Can you work these out from the model? Positions are in its coordinate system, mm. Give positions to 0.01 mm unless a question says otherwise; leave off trailing zeros. Write each loop counter-clockwise with the first axis right and the second up, starting at its lowest first coordinate (ties: lowest second). Pieces come first, ordered by that corner, then holes. Notation, with made-up numbers: (50.5, 19) -> (107.5, 19) arc R31 ccw to (107.5, 49) -> close; hole circle Ø2 at (48.5, 44.5). An arc over 180 degrees is marked (long way). One line per item, written item: value.
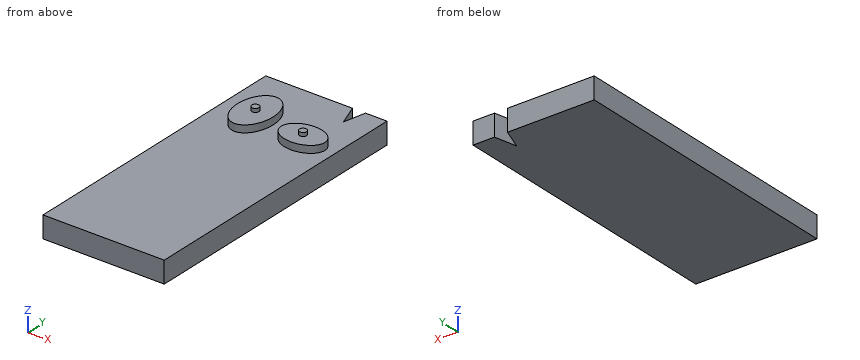
from build123d import *

# Parameters (mm, degrees)
F1_DEPTH = 3
F0_R     = 0.5
F2_DEPTH = 4
F3_DEPTH = 4.5


with BuildPart() as f1:
    # F0 (on Top) → F1 (new body)
    with BuildSketch(Plane.XY):
        Polygon((-42.22717, 54.8594), (-54.246616, 54.8594), (-54.246616, 14.957247), (-37.451323, 14.957247), (-37.451323, 54.8594), (-40.430126, 54.8594), (-41.114714, 51.767185), align=None)
        with BuildLine():
            add(Edge.make_bspline(
                [(-49.261443, 42.794443), (-44.9895, 42.794443), (-47.125472, 48.428944), (-49.261443, 54.063445), (-51.397415, 48.428944), (-53.533386, 42.794443), (-49.261443, 42.794443)],
                knots=[0, 0, 0, 2.094395, 2.094395, 4.18879, 4.18879, 6.283185, 6.283185, 6.283185], degree=2, weights=[1, 0.5, 1, 0.5, 1, 0.5, 1]))
        make_face(mode=Mode.SUBTRACT)
        with BuildLine():
            add(Edge.make_bspline(
                [(-38.755624, 45.423176), (-38.755624, 49.162015), (-43.297707, 47.292595), (-47.83979, 45.423176), (-43.297707, 43.553757), (-38.755624, 41.684338), (-38.755624, 45.423176)],
                knots=[0, 0, 0, 2.094395, 2.094395, 4.18879, 4.18879, 6.283185, 6.283185, 6.283185], degree=2, weights=[1, 0.5, 1, 0.5, 1, 0.5, 1]))
        make_face(mode=Mode.SUBTRACT)
    extrude(amount=F1_DEPTH)

    # F0 (on Top) → F2 (join)
    with BuildSketch(Plane.XY):
        with BuildLine():
            add(Edge.make_bspline(
                [(-49.261443, 42.794443), (-44.9895, 42.794443), (-47.125472, 48.428944), (-49.261443, 54.063445), (-51.397415, 48.428944), (-53.533386, 42.794443), (-49.261443, 42.794443)],
                knots=[0, 0, 0, 2.094395, 2.094395, 4.18879, 4.18879, 6.283185, 6.283185, 6.283185], degree=2, weights=[1, 0.5, 1, 0.5, 1, 0.5, 1]))
        make_face()
        with Locations((-49.261443, 46.550777)):
            Circle(F0_R, mode=Mode.SUBTRACT)
        with BuildLine():
            add(Edge.make_bspline(
                [(-38.755624, 45.423176), (-38.755624, 49.162015), (-43.297707, 47.292595), (-47.83979, 45.423176), (-43.297707, 43.553757), (-38.755624, 41.684338), (-38.755624, 45.423176)],
                knots=[0, 0, 0, 2.094395, 2.094395, 4.18879, 4.18879, 6.283185, 6.283185, 6.283185], degree=2, weights=[1, 0.5, 1, 0.5, 1, 0.5, 1]))
        make_face()
        with Locations((-41.783679, 45.423176)):
            Circle(F0_R, mode=Mode.SUBTRACT)
    extrude(amount=F2_DEPTH)

    # F0 (on Top) → F3 (join)
    with BuildSketch(Plane.XY):
        with Locations((-49.261443, 46.550777)):
            Circle(F0_R)
        with Locations((-41.783679, 45.423176)):
            Circle(F0_R)
    extrude(amount=F3_DEPTH)


solid = f1.part
1) If we section it at A-A (x = -52.25): Write out the boundary of the cut face in (y, z).
Answer list:
outline: (14.96, 0) -> (54.86, 0) -> (54.86, 3) -> (14.96, 3) -> close
2) Will these pins go through, and if not, where does the flat tip stop? pin 1 (8.5 mm diameter, centred on x = -45.5, y = 39.5, fed in from +Z); pin 2 (3 mm diameter, centred on x = -41, y = 24, fed in from -Z).
Answer list:
pin 1: stops at z = 3
pin 2: stops at z = 0
3) If we section it at B-B (y = 40.5): Write out the boundary of the cut face in (x, z), and give its area (3 significant figures).
Answer list:
outline: (-54.25, 0) -> (-37.45, 0) -> (-37.45, 3) -> (-54.25, 3) -> close
area: 50.4 mm^2
4) I need wall thicknesses on L1, parallel to Z at x = -41.5, y = 20; L2, parallel to Y at x = -47.25, z = 3.1; L3, parallel to Y at x = -44.25, z = 3.7. Which ranges of each line are inside material? Lowest first, please.
Answer list:
L1: z = 0 to 3
L2: y = 44.38 to 48.72
L3: y = 44.17 to 46.68
